from build123d import *

# Parameters (mm, degrees)
SKETCH2_W          = 2
SKETCH2_H          = 29.895029915
CUT_EXTRUDE1_DEPTH = 2


with BuildPart() as part:
    # Sketch1 → Base-Revolve (revolve)
    with BuildSketch(Plane.XY):
        Polygon((0, 11.5), (-4.5, 11.5), (-4.5, 14.5), (-1.721687836, 14.5), (-1, 13.25), (0, 13.25), align=None)
    revolve(axis=Axis((0, 0, 0), (-1, 0, 0)))

    # Sketch2 → Cut-Extrude1 (cut)
    with BuildSketch(Plane.ZY.offset(4.5)):
        with Locations((0, -0.110232412)):
            Rectangle(SKETCH2_W, SKETCH2_H)
    extrude(amount=-CUT_EXTRUDE1_DEPTH, mode=Mode.SUBTRACT)


solid = part.part
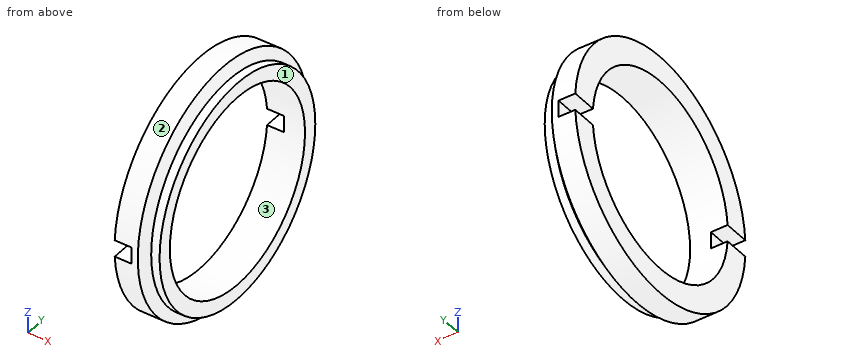
Geometry check sheet. Reference: the model listing, model coordinates, mm. Face numbers are marked on the shaded views. Give positions to 0.01 mm unless a question says otherwise; leave off trailing zeros. Loops run counter-clockwise (first coordinate to the right, second up) from the corner with the lowest first, then second, coordinate; pieces in that order, holes last.
(1) Section check B-B on y = 0. Record the cut outline in (x, z).
From the geometry:
outline: (-4.5, -14.5) - (-1.72, -14.5) - (-1, -13.25) - (0, -13.25) - (0, -11.5) - (-4.5, -11.5) - close; (-4.5, 11.5) - (0, 11.5) - (0, 13.25) - (-1, 13.25) - (-1.72, 14.5) - (-4.5, 14.5) - close
(2) Thickness scan on L1, parallel to Z at x = -3.45, y = -1; L2, parallel to Z at x = -2.7, y = -7.5; L3, parallel to Y at x = -3.6, z = -7.25. Record the ranges inside material, lowest first.
From the geometry:
L1: z = -14.47 to -11.46, 11.46 to 14.47
L2: z = -12.41 to -8.72, 8.72 to 12.41
L3: y = -12.56 to -8.93, 8.93 to 12.56
(3) Release check for a two-part mould opening along Z. For the marked faces 1, 2 and 3 record: released by +Z, released by -Z, zero draft, split by the parting line, or undercut.
From the geometry:
face 1: zero draft
face 2: split by the parting line
face 3: undercut
(4) Section check A-A on z = 0. Record the cut outline in (x, y), then the cut area to 3 significant figures.
From the geometry:
outline: (-2.5, -14.5) - (-1.72, -14.5) - (-1, -13.25) - (0, -13.25) - (0, -11.5) - (-2.5, -11.5) - close; (-2.5, 11.5) - (0, 11.5) - (0, 13.25) - (-1, 13.25) - (-1.72, 14.5) - (-2.5, 14.5) - close
area: 11.6 mm2
(5) Section check C-C on x = -2.95. Record the cut outline in (y, z), then the cut area to 3 significant figures.
From the geometry:
outline: (-14.47, -1) arc R14.5 ccw to (14.47, -1) - (11.46, -1) arc R11.5 cw to (-11.46, -1) - close; (-14.47, 1) - (-11.46, 1) arc R11.5 cw to (11.46, 1) - (14.47, 1) arc R14.5 ccw to start
area: 233 mm2
(6) Depth check by flat-ended pin: pin 1 Ø0.6 at (y, z) = (13.5, 0) entering from -X; pin 2 Ø1.6 at (x, y) = (-3.5, 12.5) entering from +Z; pin 3 Ø1 at (x, y) = (-4, -13.5) entering from -Z. Enter the tip coordinate at first touch or a pass-through.
From the geometry:
pin 1: stops at x = -2.5
pin 2: stops at z = 8.57
pin 3: stops at z = -6.42
